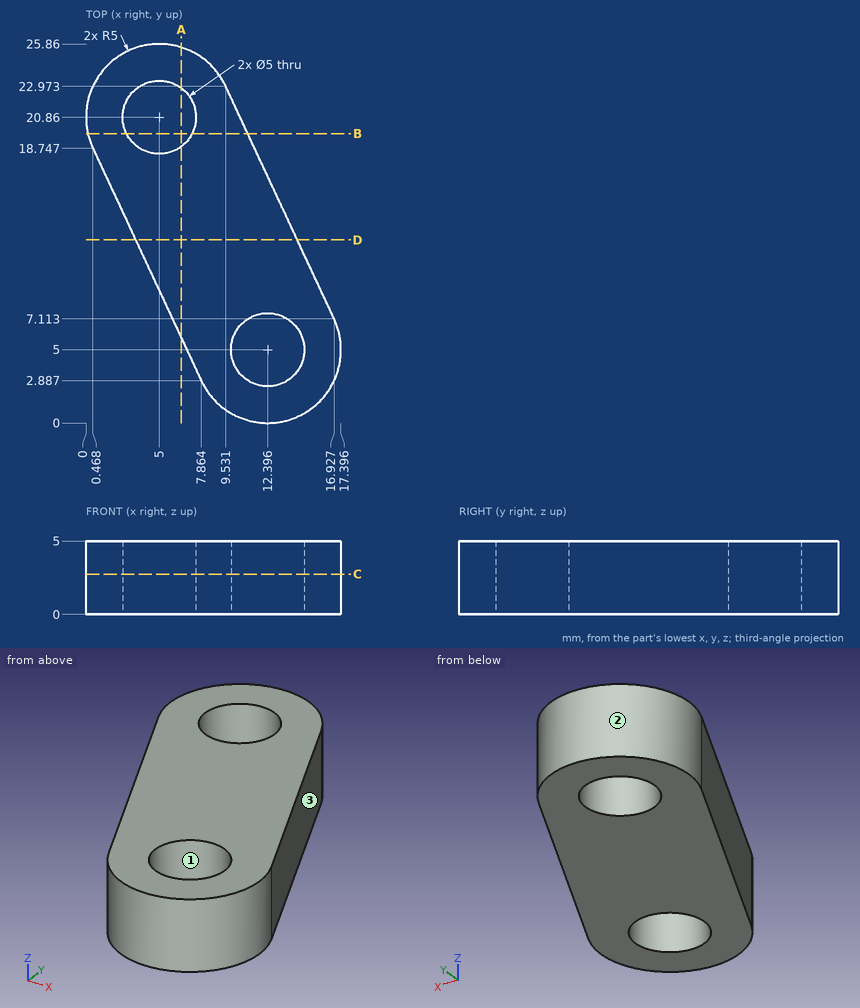
Can you work these out from the drawing? Everything is in mm from the part's minimum corner. Coordinates: 2 decimals unless noted, no trailing zeros. Loops run counter-clockwise (first coordinate to the right, second up) from the corner with the lowest first, then second, coordinate; pieces in that order, holes last. Notation, with made-up numbers: M -16.75,69 L 41.25,69 A29 ccw 41.25,99 Z; hole C 24.25,83.5 d9. An arc over 180 degrees is marked long. One line per item, written item: value.
1. Imagine slicing it at B-B (y = 19.75). List the corners of the cut face in (x, z) for me (1 decimal).
Geometry says:
outline: M 0.1,0 L 2.8,0 L 2.8,5 L 0.1,5 Z; M 7.2,0 L 11,0 L 11,5 L 7.2,5 Z
2. Imagine slicing it at A-A (x = 6.5). List the corners of the cut face in (y, z) for me.
Geometry says:
outline: M 5.81,0 L 18.86,0 L 18.86,5 L 5.81,5 Z; M 22.86,0 L 25.63,0 L 25.63,5 L 22.86,5 Z
3. Thinking about a two-plate mould opening in Y: for the marked faces 1, 2 and 3, which applies, +Y half, -Y half, draft (parallel to the pull), parting line (faces both ways), or undercut?
Geometry says:
face 1: undercut
face 2: parting line
face 3: +Y half
4. Will these pins go through, and if not, where does the flat tip stop? pin 1 Ø1 at (x, z) = (15, 2.5) entering from +Y; pin 2 Ø3 at (x, z) = (2.5, 4.5) entering from -Y (1 decimal); pin 3 Ø1 at (x, z) = (13, 1.5) entering from +Y (1 decimal).
Geometry says:
pin 1: stops at y = 12.32
pin 2: stops at y = 11.2
pin 3: stops at y = 16.6
5. Imagine slicing it at C-C (z = 2.75). List the corners of the cut face in (x, y) for me (1 decimal), and give its area (3 significant figures).
Geometry says:
outline: M 0.5,18.7 L 7.9,2.9 A5 ccw 16.9,7.1 L 9.5,23 A5 ccw Z; hole C 5,20.9 d5; hole C 12.4,5 d5
area: 214 mm2
6. Imagine slicing it at D-D (y = 12.5). List the corners of the cut face in (x, z) for me (1 decimal).
Geometry says:
outline: M 3.4,0 L 14.4,0 L 14.4,5 L 3.4,5 Z
7. Please list where these lines run through material, in increasing order: probe 1 along X at (y, z) = (18.75, 2.15) (1 decimal); probe 2 along Y at (x, z) = (5, 2.5) (1 decimal); probe 3 along Y at (x, z) = (6.5, 2.35) (1 decimal).
Geometry says:
probe 1: x = 0.5 to 3.7, 6.3 to 11.5
probe 2: y = 9 to 18.4, 23.4 to 25.9
probe 3: y = 5.8 to 18.9, 22.9 to 25.6
